from build123d import *

# Parameters (mm, degrees)
SKETCH1_W                      = 63.246
SKETCH1_H                      = 36.83
EXTRUDE1_DEPTH                 = 25.4
M4X0_7_TAPPED_HOLE1_AT_2_COUNT = 2
M4X0_7_TAPPED_HOLE1_AT_2_PITCH = 17.517255065
M4X0_7_TAPPED_HOLE2_AT_2_COUNT = 2
M4X0_7_TAPPED_HOLE2_AT_2_PITCH = 17.517255065
SKETCH6_W                      = 29.464
SKETCH6_H                      = 36.83
EXTRUDE2_DEPTH                 = 5.842
CHAMFER1_SIZE                  = 5.842
CHAMFER2_SIZE                  = 5.842
CHAMFER3_SIZE2                 = 5.842
CHAMFER3_SIZE                  = 10
SKETCH7_R                      = 2.97815
EXTRUDE3_DEPTH                 = 18.5801


with BuildPart() as part:
    # Sketch1 → Extrude1 (new body)
    with BuildSketch(Plane.XY):
        with Locations((31.623, 18.415)):
            Rectangle(SKETCH1_W, SKETCH1_H)
    extrude(amount=EXTRUDE1_DEPTH)

    # Sketch2 → M4x0.7 Tapped Hole1 (revolve, cut)
    with BuildSketch(Plane(origin=(37.846, 0, 6.6675), x_dir=(0, 0, -1), z_dir=(1, 0, 0))):
        Polygon((0, 0), (0, 6.071420021), (1.65, 5.08), (1.65, 8.0000094), (2, 8.0000094), (2, 0), align=None)
    m4x0_7_tapped_hole1 = revolve(axis=Axis((37.846, -6.35, 6.6675), (0, 1, 0)), mode=Mode.SUBTRACT)

    # M4x0.7 Tapped Hole1 at 2: M4x0.7 Tapped Hole1 ×2
    with Locations(*[Vector(0.7249994335944138, 0, 0.6887494619146932) * (i * M4X0_7_TAPPED_HOLE1_AT_2_PITCH) for i in range(1, M4X0_7_TAPPED_HOLE1_AT_2_COUNT)]):
        add(m4x0_7_tapped_hole1, mode=Mode.SUBTRACT)

    # Sketch5 → M4x0.7 Tapped Hole2 (revolve, cut)
    with BuildSketch(Plane(origin=(50.546, 36.83, 6.6675), x_dir=(0, 0, 1), z_dir=(1, 0, 0))):
        Polygon((0, 0), (0, 6.071420021), (1.65, 5.08), (1.65, 8.0000094), (2, 8.0000094), (2, 0), align=None)
    m4x0_7_tapped_hole2 = revolve(axis=Axis((50.546, 43.18, 6.6675), (0, -1, 0)), mode=Mode.SUBTRACT)

    # M4x0.7 Tapped Hole2 at 2: M4x0.7 Tapped Hole2 ×2
    with Locations(*[Vector(-0.7249994335944137, 0, 0.6887494619146932) * (i * M4X0_7_TAPPED_HOLE2_AT_2_PITCH) for i in range(1, M4X0_7_TAPPED_HOLE2_AT_2_COUNT)]):
        add(m4x0_7_tapped_hole2, mode=Mode.SUBTRACT)

    # Sketch6 → Extrude2 (add)
    with BuildSketch(Plane.XY.offset(25.4)):
        with Locations((24.892, 18.415)):
            Rectangle(SKETCH6_W, SKETCH6_H)
    extrude(amount=EXTRUDE2_DEPTH)

    # Chamfer1
    chamfer1_edges = [part.edges().sort_by_distance(p)[0] for p in [
        (24.892, 0, 31.242),
    ]]
    chamfer(chamfer1_edges, length=CHAMFER1_SIZE)

    # Chamfer2
    chamfer2_edges = [part.edges().sort_by_distance(p)[0] for p in [
        (24.892, 36.83, 31.242),
    ]]
    chamfer(chamfer2_edges, length=CHAMFER2_SIZE)

    # Chamfer3
    chamfer3_edges = [part.edges().sort_by_distance(p)[0] for p in [
        (39.624, 18.415, 31.242),
    ]]
    chamfer3_side = [part.faces().sort_by_distance(p)[0] for p in [
        (39.50716, 18.415, 31.242),
    ]]
    chamfer(chamfer3_edges, length=CHAMFER3_SIZE - 0.0001, length2=CHAMFER3_SIZE2 - 0.0001, reference=chamfer3_side[0])  # a hair under: the kernel refuses the full size

    # Sketch7 → Extrude3 (add)
    with BuildSketch(Plane.ZY):
        with Locations(Location((12.7, 28.956, 0), (0, 0, 180))):
            Circle(SKETCH7_R)
        with Locations(Location((12.7, 7.874, 0), (0, 0, 180))):
            Circle(SKETCH7_R)
    extrude(amount=EXTRUDE3_DEPTH)


solid = part.part
Can you work these out from the model? Positions are in its coordinate system, mm. A direction names the side the tool comes from. Give positions to 0.01 mm unless a question says otherwise; leave off trailing zeros. Order: outer loops, then holes, each group sorted by start corner. A loop starts at its lowest first (then second) coordinate and runs counter-clockwise, first axis right, second up. Notation, with made-up numbers: M -15.5,62 L 41.5,62 A12 cw 41.5,73 Z; hole C 34,-31.75 d7. An arc over 180 degrees is marked long. Use one line per item in the form item = value. Start each with the question number.
Item 1: We'd pull the mould along X, two halves only. Please class faces 4 (the cylindrical face through (48.86, 3.94, 17.66)), 5 (the cylindrical face through (-9.16, 9.015, 9.949)), 6 (the flat face through (0, 18, 13)): +X half, -X half, draft (parallel to the pull), parting line (faces both ways), or undercut.
Item 2: Will these pins go through, and if not, where does the flat tip stop? pin 1 Ø3 at (x, y) = (4.5, 27.5) entering from +Z; pin 2 Ø2 at (x, y) = (-4, 29) entering from +Z; pin 3 Ø1.2 at (x, z) = (37, 19.5) entering from +Y.
Item 3: If we section it at A-A (x = 24): Write out the boundary of the cut face in (y, z), then the cut area to 3 significant figures.
Item 4: If I drill on line 1 along X through (y, z) = (25.5, 9.5); line 2 along Z through (x, y) = (44.5, 17.5); line 3 along Y through (x, z) = (50.5, 20.5), over which ranges is the centre line in solid material (lowest first)?
Item 5: For faces 1 (the flat face through (10.16, 18, 28)), 2 (the cylindrical face through (36.16, 32.89, 19.81)), 3 (the cylindrical face through (39.8, 3.9, 7.1)), which set-ups out of +Z, -Z, +X, -X, +Y, -Y let a thin tool reach every point of the face, with its end or its side?
Item 6: If we section it at C-C (z = 12.7): Write out the boundary of the cut face in (x, y).
Outcome:
q1.face_4 = undercut
q1.face_5 = draft
q1.face_6 = -X half
q2.pin_1 = 25.4
q2.pin_2 = 15.68
q2.pin_3 = 31.75
q3.outline = M 0,0 L 36.83,0 L 36.83,25.4 L 30.99,31.24 L 5.84,31.24 L 0,25.4 Z
q3.area = 1,120 mm2
q4.line_1 = 0 to 63.25
q4.line_2 = 0 to 25.4
q4.line_3 = 8 to 36.83
q5.face_1 = +Z, -X, +Y, -Y
q5.face_2 = +Y
q5.face_3 = -Y
q6.outline = M -18.58,4.9 L 0,4.9 L 0,0 L 63.25,0 L 63.25,36.83 L 0,36.83 L 0,31.93 L -18.58,31.93 L -18.58,25.98 L 0,25.98 L 0,10.85 L -18.58,10.85 Z
